Model file for the job. Use its own axes, mm. Coordinates: 2 decimals unless noted, no trailing zeros. Write each loop counter-clockwise with the first axis right and the second up, starting at its lowest first coordinate (ties: lowest second). Pieces come first, ordered by that corner, then holes. Notation, with made-up numbers: M -21.5,73.25 L 31.5,73.25 A35 ccw 31.5,105.25 Z; hole C 48,85.5 d5. An arc over 180 degrees is marked long. Use CSV: the item, a comma, the result in double quotes. Start each with the question number.
from build123d import *

# Parameters (mm, degrees)
SKETCH2_W           = 84.57
SKETCH2_H           = 90.8
BOSS_EXTRUDE1_DEPTH = 1.6
SKETCH3_R           = 1.5
CUT_EXTRUDE1_DEPTH  = 2.6
SKETCH4_W           = 90.8
SKETCH4_H           = 1.6
BOSS_EXTRUDE2_DEPTH = 2.88
SKETCH5_W           = 90.8
SKETCH5_H           = 1.6
BOSS_EXTRUDE3_DEPTH = 2.59
SKETCH6_W           = 90.04
SKETCH6_H           = 1.6
BOSS_EXTRUDE4_DEPTH = 2.54
SKETCH7_W           = 90.04
SKETCH7_H           = 1.6
BOSS_EXTRUDE5_DEPTH = 2.54


with BuildPart() as part:
    # Sketch2 → Boss-Extrude1 (new body)
    with BuildSketch(Plane(origin=(0, 0, 0), x_dir=(1, 0, 0), z_dir=(0, 1, 0))):
        with Locations((42.285, 45.4)):
            Rectangle(SKETCH2_W, SKETCH2_H)
    extrude(amount=BOSS_EXTRUDE1_DEPTH)

    # Sketch3 → Cut-Extrude1 (cut, through all)
    with BuildSketch(Plane(origin=(0, 1.6, 0), x_dir=(1, 0, 0), z_dir=(0, 1, 0))):
        with Locations((2.5, 2.5)):
            Circle(SKETCH3_R)
        with Locations((82.07, 2.5)):
            Circle(SKETCH3_R)
        with Locations((5.8, 88.3)):
            Circle(SKETCH3_R)
        with Locations((79.37, 88.3)):
            Circle(SKETCH3_R)
    extrude(amount=-CUT_EXTRUDE1_DEPTH, mode=Mode.SUBTRACT)

    # Sketch4 → Boss-Extrude2 (add)
    with BuildSketch(Plane(origin=(84.57, 0, 0), x_dir=(0, 0, -1), z_dir=(1, 0, 0))):
        with Locations((45.4, 0.8)):
            Rectangle(SKETCH4_W, SKETCH4_H)
    extrude(amount=BOSS_EXTRUDE2_DEPTH)

    # Sketch5 → Boss-Extrude3 (add)
    with BuildSketch(Plane.ZY):
        with Locations((-45.4, 0.8)):
            Rectangle(SKETCH5_W, SKETCH5_H)
    extrude(amount=BOSS_EXTRUDE3_DEPTH)

    # Sketch6 → Boss-Extrude4 (add)
    with BuildSketch(Plane(origin=(0, 0, -90.8), x_dir=(-1, 0, 0), z_dir=(0, 0, -1))):
        with Locations((-42.43, 0.8)):
            Rectangle(SKETCH6_W, SKETCH6_H)
    extrude(amount=BOSS_EXTRUDE4_DEPTH)

    # Sketch7 → Boss-Extrude5 (add)
    with BuildSketch(Plane.XY):
        with Locations((42.43, 0.8)):
            Rectangle(SKETCH7_W, SKETCH7_H)
    extrude(amount=BOSS_EXTRUDE5_DEPTH)


solid = part.part
1) Band-saw the part on B-B on z = -88.3. List the corners of the cut face in (x, y), then the cut area to 3 significant figures.
2) Wall check: L1, parallel to X at y = 0.75, z = -88.3; L2, parallel to X at y = 0.4, z = -2.5; L3, parallel to Z at x = 5.8, y = 1.2. Give the ranges that are in metal, low to high. Write a range as [from, to].
3) Two-plate mould, pull along Z, no slides. Class faces 1 (the face through (42, 0, -46)), 2 (the face through (79.045, 0.811, -86.836)): pulls with the +Z half, pulls with the -Z half, needs draft (parallel to the pull), parting line crosses it, or undercut.
4) Band-saw the part on A-A on x = 2.5. List the corners of the cut face in (y, z).
5) Drop flat-ended pins along their axis: P1, Ø2.5, axis at x = 79.37, z = -88.3, coming from the +Y side; P2, Ø4, axis at x = 2.5, z = -2.5, coming from the +Y side. Give the stop position or say it passes through.
Findings below:
1,outline,"M -2.59,0 L 4.3,0 L 4.3,1.6 L -2.59,1.6 Z; M 7.3,0 L 77.87,0 L 77.87,1.6 L 7.3,1.6 Z; M 80.87,0 L 87.45,0 L 87.45,1.6 L 80.87,1.6 Z"
1,area,"134 mm2"
2,L1,"x = [-2.59, 4.3], [7.3, 77.87], [80.87, 87.45]"
2,L2,"x = [-2.59, 1], [4, 80.57], [83.57, 87.45]"
2,L3,"z = [-93.34, -89.8], [-86.8, 2.54]"
3,face 1,"needs draft"
3,face 2,"undercut"
4,outline,"M 0,-93.34 L 1.6,-93.34 L 1.6,-4 L 0,-4 Z; M 0,-1 L 1.6,-1 L 1.6,2.54 L 0,2.54 Z"
5,P1,"passes through"
5,P2,"stops at y = 1.6"
